Verification items for the finished model (mm, model axes). A direction names the side the tool comes from. Coordinates: 2 decimals unless noted, no trailing zeros. Write each loop counter-clockwise with the first axis right and the second up, starting at its lowest first coordinate (ties: lowest second). Pieces come first, ordered by that corner, then holes. Notation, with made-up numbers: M 11,5 L 57,5 A28 ccw 57,38 Z; hole C 4.5,18.5 d6. An arc over 180 degrees is marked long. Answer in a Markdown table with one row per item.
from build123d import *

# Parameters (mm, degrees)
SKETCH_1_R          = 10
EXTRUDE_1_DEPTH     = 16
SKETCH_2_R          = 2
CUT_EXTRUDE_1_DEPTH = 10
SKETCH_4_R          = 8.4
CUT_EXTRUDE_2_DEPTH = 1
SKETCH_5_R          = 3.93
EXTRUDE_2_DEPTH     = 1


with BuildPart() as part:
    # 草图1 → 凸台-拉伸1 (new body)
    with BuildSketch(Plane(origin=(0, 0, 0), x_dir=(0, 0, -1), z_dir=(1, 0, 0))):
        Circle(SKETCH_1_R)
    extrude(amount=EXTRUDE_1_DEPTH)

    # 草图2 → 切除-拉伸1 (cut)
    with BuildSketch(Plane(origin=(16, 0, 0), x_dir=(0, 0, -1), z_dir=(1, 0, 0))):
        Circle(SKETCH_2_R)
    extrude(amount=-CUT_EXTRUDE_1_DEPTH, mode=Mode.SUBTRACT)

    # 草图4 → 切除-拉伸2 (cut)
    with BuildSketch(Plane.ZY):
        Circle(SKETCH_4_R)
    extrude(amount=-CUT_EXTRUDE_2_DEPTH, mode=Mode.SUBTRACT)

    # 草图5 → 凸台-拉伸2 (add)
    with BuildSketch(Plane.ZY.offset(-1)):
        Circle(SKETCH_5_R)
    extrude(amount=EXTRUDE_2_DEPTH)


solid = part.part
1) Release check for a two-part mould opening along Z. For faces 4 (the face through (7.89, -9.76, 2.17)), 5 (the face through (0, 7, 5)), 6 (the face through (1, -2, 4)) record: +Z half, -Z half, draft (parallel to the pull), parting line (faces both ways), or undercut.
Response values:
| item | result |
|---|---|
| face 4 | parting line |
| face 5 | draft |
| face 6 | undercut |
2) Sectioned sample at B-B (z = 3). Record the cut outline in (x, y).
Response values:
| item | result |
|---|---|
| outline | M 0,-9.54 L 16,-9.54 L 16,9.54 L 0,9.54 L 0,7.85 L 1,7.85 L 1,2.54 L 0,2.54 L 0,-2.54 L 1,-2.54 L 1,-7.85 L 0,-7.85 Z |
3) Thickness scan on L1, parallel to Y at x = 0.4, z = 0; L2, parallel to Y at x = 13, z = 0; L3, parallel to X at y = -3.5, z = -3.5. Record the ranges inside material, lowest first. Write a range as [from, to].
Response values:
| item | result |
|---|---|
| L1 | y = [-10, -8.4], [-3.93, 3.93], [8.4, 10] |
| L2 | y = [-10, -2], [2, 10] |
| L3 | x = [1, 16] |
4) Depth check by flat-ended pin: pin 1 (4 mm diameter, centred on x = 7.5, y = -4, fed in from -Z); pin 2 (1.5 mm diameter, centred on x = 11.5, z = 1, fed in from +Y); pin 3 (3 mm diameter, centred on x = 4, z = -6, fed in from +Y). Enter the tip coordinate at first touch or a pass-through.
Response values:
| item | result |
|---|---|
| pin 1 | stops at z = -9.8 |
| pin 2 | stops at y = 10 |
| pin 3 | stops at y = 8.93 |
5) Sectioned sample at A-A (y = 0). Record the cut outline in (x, z).
Response values:
| item | result |
|---|---|
| outline | M 0,-10 L 16,-10 L 16,-2 L 6,-2 L 6,2 L 16,2 L 16,10 L 0,10 L 0,8.4 L 1,8.4 L 1,3.93 L 0,3.93 L 0,-3.93 L 1,-3.93 L 1,-8.4 L 0,-8.4 Z |
6) Tool access check on faces 1 (the face through (0.507, -3.837, -0.852)), 2 (the face through (0, 0, 0)), 3 (the face through (6, 0, 0)). Record the directions out of +Z, -Z, +X, -X, +Y, -Y that give a thin tool (end or side, any length) a straight path to the whole face; none if there is none.
Response values:
| item | result |
|---|---|
| face 1 | -X |
| face 2 | +Z, -Z, -X, +Y, -Y |
| face 3 | +X |
7) Sectioned sample at C-C (x = 10.75). Record the cut outline in (y, z), then the cut area to 3 significant figures.
Response values:
| item | result |
|---|---|
| outline | C 0,0 d20; hole C 0,0 d4 |
| area | 302 mm² |
8) Sectioned sample at D-D (x = 5.5). Record the cut outline in (y, z), then the cut area to 3 significant figures.
Response values:
| item | result |
|---|---|
| outline | C 0,0 d20 |
| area | 314 mm² |
